Verification items for the finished model (mm, model axes). A direction names the side the tool comes from. Give positions to 0.01 mm unless a question says otherwise; leave off trailing zeros. Order: outer loops, then holes, each group sorted by start corner. A loop starts at its lowest first (then second) coordinate and runs counter-clockwise, first axis right, second up.
(1) Sectioned sample at B-B on z = 41. Record the cut outline in (x, y).
(2) Sectioned sample at C-C on y = -17. Record the cut outline in (x, z).
(3) Sectioned sample at A-A on x = -13. Record the cut outline in (y, z).
(4) Scan lines: L1, parallel to Y at x = -7.5, z = -26; L2, parallel to Y at x = 0.5, z = -45.5; L3, parallel to X at y = 15.5, z = -9.5. Record each from-to range of solid material in increasing order.
(5) Access from +Z, -Z, +X, -X, +Y, -Y to the whole of each face (thin tool, end or side, straight path). Record for faces 1 (the face through (-30, 0, 1)), 2 (the face through (-16, 15, 1)), 3 (the face through (0, -20, 2.5)), 4 (the face through (16, 15, 1)), 5 (the face through (0, -15, -26)).
(6) Gauge pin test, flat ends, axial feed: pin 1 (14 mm diameter, centred on x = -23, z = -17.5, fed in from +Y); pin 2 (3 mm diameter, centred on y = 18, z = 14, fed in from -X); pin 3 (5 mm diameter, centred on x = 24, z = -34, fed in from -Y). Record the tip position at first contact, or that the pin passes through.
Autodesk Inventor part; units mm, degrees
ref_plane "YZ Plane" through (0, 0, 0) normal (1, 0, 0) x (0, 1, 0)
ref_plane "XZ Plane" through (0, 0, 0) normal (0, 1, 0) x (-1, 0, 0)
ref_plane "XY Plane" through (0, 0, 0) normal (0, 0, 1) x (1, 0, 0)
sketch "草图3" plane through (0, 0, 0) normal (0, 1, 0) x (-1, 0, 0)
  line L0 (-30, 50) -> (30, 50)
  line L1 (30, 50) -> (30, -50)
  line L2 (30, -50) -> (-30, -50)
  line L3 (-30, -50) -> (-30, 50)
  line L4 (-30, 50) -> (30, -50) construction
  line L5 (30, 50) -> (-30, -50) construction
  point P0 (0, 0)
  dimension "d21" = 60
  dimension "d22" = 100
extrude "拉伸3" add sketch "草图3" against normal mid plane 30
sketch "草图4" plane through (0, 15, 0) normal (0, 1, 0) x (1, 0, 0)
  line L0 (-30, -50) -> (-2.5, -50)
  line L1 (30, -50) -> (-30, -50)
  line L2 (-2.5, -50) -> (-2.5, 50)
  line L3 (-2.5, 50) -> (2.5, 50)
  line L4 (-30, 50) -> (30, 50)
  line L5 (2.5, 50) -> (2.5, -50)
  line L6 (2.5, -50) -> (-2.5, -50)
  point P0 (0, 0)
  point P1 (2.5, -50)
  dimension "d25" = 27.5
  dimension "d31" = 5
extrude "拉伸4" add sketch "草图4" along normal blind 10
sketch "草图5" plane through (0, -15, 0) normal (0, -1, 0) x (1, 0, 0)
  line L0 (30, 50) -> (30, -50)
  line L1 (-30, 2.5) -> (30, 2.5)
  line L2 (30, 2.5) -> (30, -2.5)
  line L3 (30, -2.5) -> (-30, -2.5)
  line L4 (-30, -2.5) -> (-30, 2.5)
  line L5 (-30, 2.5) -> (30, -2.5) construction
  line L6 (30, 2.5) -> (-30, -2.5) construction
  point P0 (0, 0)
  dimension "d28" = 5
extrude "拉伸5" add sketch "草图5" along normal blind 10
properties part number "水平滑盖"
Ans:
1. outline: (-30, -15) - (30, -15) - (30, 15) - (2.5, 15) - (2.5, 25) - (-2.5, 25) - (-2.5, 15) - (-30, 15) - close
2. outline: (-30, -2.5) - (30, -2.5) - (30, 2.5) - (-30, 2.5) - close
3. outline: (-25, -2.5) - (-15, -2.5) - (-15, -50) - (15, -50) - (15, 50) - (-15, 50) - (-15, 2.5) - (-25, 2.5) - close
4. L1: y = -15 to 15
4. L2: y = -15 to 25
4. L3: x = -2.5 to 2.5
5. face 1: +Z, -Z, -X, +Y, -Y
5. face 2: +Z, -Z, -X, +Y
5. face 3: +Z, +X, -X, -Y
5. face 4: +Z, -Z, +X, +Y
5. face 5: -Z, +X, -X, -Y
6. pin 1: stops at y = 15
6. pin 2: stops at x = -2.5
6. pin 3: stops at y = -15
